For this review, take the finished solid that the model builds, in its own axes (mm). A direction names the side the tool comes from. Round coordinates to 2 decimals unless told otherwise and drop trailing zeros. Loops run counter-clockwise (first coordinate to the right, second up) from the corner with the lowest first, then second, coordinate; pieces in that order, holes last.
1) Insertion check: pin 1 (4 mm diameter, centred on y = -73, z = -3.5, fed in from -X); pin 2 (4 mm diameter, centred on x = 2.5, z = 14.5, fed in from -Y); pin 3 (12 mm diameter, centred on x = 0.5, y = -82.5, fed in from -Z). Each pin has a flat end and moves straight along its axis. Give the tip position at first contact, or say it passes through.
2) Take a section at A-A (x = 0). State the section outline as (y, z) points (1 decimal), then the cut area to 3 significant figures.
3) Take a section at B-B (z = 0). State the section outline as (x, y) points (1 decimal), then the cut area to 3 significant figures.
4) Take a section at C-C (y = -14.5). State the section outline as (x, z) points.
5) Tool access review of faces 1 (the cylindrical face through (-2.343, -27.368, 17.847)), 2 (the cylindrical face through (-3.47, -73.96, -15.62)): name each direction out of +Z, -Z, +X, -X, +Y, -Y from which nothing blocks a thin tool from reaching the whole face with its end or side.
6) Wall thickness on L1, parallel to Y at x = 8, z = -9; L2, parallel to X at y = -75.5, z = -5; L3, parallel to X at y = -10, z = 10.5: over which ranges is each line inside the solid? List them lowest first.
```python
from build123d import *

# Parameters (mm, degrees)
F0_R     = 18
F1_DEPTH = 57.1
F2_R     = 16
F3_DEPTH = 35
F4_R     = 1.5875
F5_R     = 3
F6_DEPTH = 19.3
F7_SIZE  = 0.79375


with BuildPart() as f1:
    # F0 (on Front) → F1 (new body)
    with BuildSketch(Plane.XZ):
        Circle(F0_R)
    extrude(amount=F1_DEPTH)

    # F2 (on face) → F3 (join)
    with BuildSketch(Plane.XZ.offset(57.1)):
        Circle(F2_R)
    extrude(amount=F3_DEPTH)

    # F4
    f4_edges = [f1.edges().sort_by_distance(p)[0] for p in [
        (-18, -57.1, 0),
    ]]
    fillet(f4_edges, radius=F4_R)

    # F5 (on face) → F6 (join)
    with BuildSketch(Plane.XZ.offset(92.1)):
        Circle(F5_R)
    extrude(amount=F6_DEPTH)

    # F7
    f7_edges = [f1.edges().sort_by_distance(p)[0] for p in [
        (-16, -92.1, 0),
    ]]
    chamfer(f7_edges, length=F7_SIZE)


solid = f1.part
```
Response:
1. pin 1: stops at x = -15.93
1. pin 2: stops at y = -92.1
1. pin 3: stops at z = -16
2. outline: (-111.4, -3) - (-92.1, -3) - (-92.1, -15.2) - (-91.3, -16) - (-57.1, -16) - (-57.1, -16.4) arc R1.6 ccw to (-55.5, -18) - (0, -18) - (0, 18) - (-55.5, 18) arc R1.6 ccw to (-57.1, 16.4) - (-57.1, 16) - (-91.3, 16) - (-92.1, 15.2) - (-92.1, 3) - (-111.4, 3) - close
2. area: 3,290 mm2
3. outline: (-18, -55.5) arc R1.6 ccw to (-16.4, -57.1) - (-16, -57.1) - (-16, -91.3) - (-15.2, -92.1) - (-3, -92.1) - (-3, -111.4) - (3, -111.4) - (3, -92.1) - (15.2, -92.1) - (16, -91.3) - (16, -57.1) - (16.4, -57.1) arc R1.6 ccw to (18, -55.5) - (18, 0) - (-18, 0) - close
3. area: 3,290 mm2
4. outline: circle Ø36 at (0, 0)
5. face 1: +Y, -Y
5. face 2: -Y
6. L1: y = -92.1 to 0
6. L2: x = -15.2 to 15.2
6. L3: x = -14.62 to 14.62
